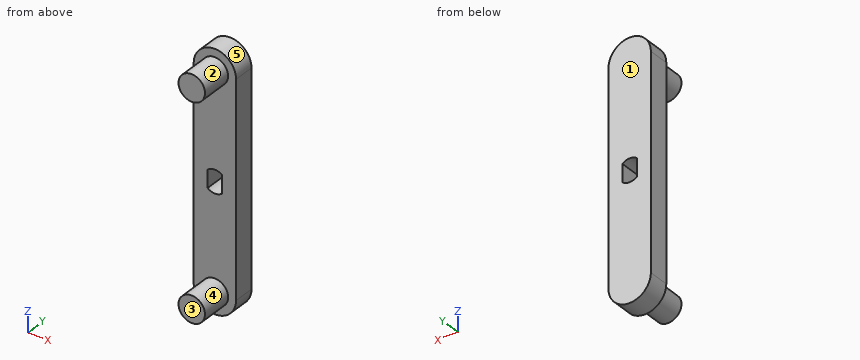
```python
from build123d import *

# Parameters (mm, degrees)
BOSS_EXTRUDE1_DEPTH = 5.08
SKETCH3_R           = 3.175
BOSS_EXTRUDE2_DEPTH = 7.62
CUT_EXTRUDE1_REACH  = 35.408


with BuildPart() as part:
    # Sketch2 → Boss-Extrude1 (new body)
    with BuildSketch(Plane(origin=(0, 0, 0), x_dir=(1, 0, 0), z_dir=(0, 1, 0))):
        with BuildLine():
            Line((-5.08, 25.4), (-5.08, -25.4))
            ThreePointArc((-5.08, -25.4), (0, -30.48), (5.08, -25.4))
            Line((5.08, -25.4), (5.08, 25.4))
            ThreePointArc((5.08, 25.4), (0, 30.48), (-5.08, 25.4))
        make_face()
    extrude(amount=BOSS_EXTRUDE1_DEPTH)

    # Sketch3 → Boss-Extrude2 (add)
    with BuildSketch(Plane(origin=(0, 0, 0), x_dir=(-1, 0, 0), z_dir=(0, -1, 0))):
        with Locations(Location((0, -25.4, 0), (0, 0, 270))):
            Circle(SKETCH3_R)
        with Locations(Location((0, 25.4, 0), (0, 0, 270))):
            Circle(SKETCH3_R)
    extrude(amount=BOSS_EXTRUDE2_DEPTH)

    # Sketch10 → Cut-Extrude1 (cut, up to next)
    with BuildSketch(Plane(origin=(0, 5.08, 0), x_dir=(1, 0, 0), z_dir=(0, 1, 0)), mode=Mode.PRIVATE) as cut_extrude1_sk1:
        with BuildLine():
            Line((-1.75, 2.121320344), (-1.75, -2.121320344))
            ThreePointArc((-1.75, -2.121320344), (0, -2.75), (1.75, -2.121320344))
            Line((1.75, -2.121320344), (1.75, 2.121320344))
            ThreePointArc((1.75, 2.121320344), (0, 2.75), (-1.75, 2.121320344))
        make_face()
    cut_extrude1_tool1 = extrude(cut_extrude1_sk1.sketch, amount=-CUT_EXTRUDE1_REACH, mode=Mode.PRIVATE) & part.part
    add(cut_extrude1_tool1.solids().sort_by_distance((0, 5.08, 0))[0], mode=Mode.SUBTRACT)


solid = part.part
```
Source: CAD feature listing. Evaluate the final solid. Frame: model axes, mm. Face numbers are marked on the shaded views. A direction names the side the tool comes from. Coordinates: 2 decimals unless noted, no trailing zeros. Write each loop counter-clockwise with the first axis right and the second up, starting at its lowest first coordinate (ties: lowest second). Pieces come first, ordered by that corner, then holes. Notation, with made-up numbers: (57, 50) -> (77, 50) arc R17 ccw to (77, 75) -> close; hole circle Ø1 at (59.25, 44). An arc over 180 degrees is marked (long way). Return JSON: item names as keys, results as strings. Group by question number.
1) Section query D-D, the plane x = 2.5. Return loops of the section in (y, z), plus the area to 3 significant figures.
2) Section query B-B, the plane y = -1. Return loops of the section in (x, z) (3 decimals).
3) Section query C-C, the plane z = 26.5. Return loops of the section in (x, y), plus the area to 3 significant figures.
4) Contact query for flat-ended pins moving along their axis: P1, Ø5, axis at x = 0, z = 7.5, coming from the -Y side; P2, Ø6, axis at x = -1.5, y = -6.5, coming from the +Z side (3 decimals). Output: stop coordinate, or through.
5) Section query A-A, the plane x = 0. Return loops of the section in (y, z) (3 decimals), plus the area to 3 significant figures.
6) Ray query, line 1 along X through (y, z) = (3.5, -2); line 2 along Y through (x, z) = (-3.75, 27.5); line 3 along Z through (x, y) = (0.25, -6.75). Return the intervals inside material, ascending.
7) Mould query, pull axis Z, two halves, no side actions, for the marked faces 3, 4 and 5. Classes: +Z half, -Z half, draft (parallel to the pull), parting line (faces both ways), or undercut.
8) Set-up query: the marked faces 1 and 2. Return all of +Z, -Z, +X, -X, +Y, -Y with unobstructed straight access to the full face (end or side cutting, diameter ignored); none if empty.
From the geometry:
{
 "1": {"outline": "(-7.62, -27.36) -> (0, -27.36) -> (0, -29.82) -> (5.08, -29.82) -> (5.08, 29.82) -> (0, 29.82) -> (0, 27.36) -> (-7.62, 27.36) -> (-7.62, 23.44) -> (0, 23.44) -> (0, -23.44) -> (-7.62, -23.44) -> close", "area": "363 mm²"},
 "2": {"outline": "circle Ø6.35 at (0, -25.4); circle Ø6.35 at (0, 25.4)"},
 "3": {"outline": "(-4.96, 0) -> (-2.98, 0) -> (-2.98, -7.62) -> (2.98, -7.62) -> (2.98, 0) -> (4.96, 0) -> (4.96, 5.08) -> (-4.96, 5.08) -> close", "area": "95.8 mm²"},
 "4": {"P1": "y = 0", "P2": "z = 28.575"},
 "5": {"outline": "(-7.62, -28.575) -> (0, -28.575) -> (0, -30.48) -> (5.08, -30.48) -> (5.08, -2.75) -> (0, -2.75) -> (0, -22.225) -> (-7.62, -22.225) -> close; (-7.62, 22.225) -> (0, 22.225) -> (0, 2.75) -> (5.08, 2.75) -> (5.08, 30.48) -> (0, 30.48) -> (0, 28.575) -> (-7.62, 28.575) -> close", "area": "379 mm²"},
 "6": {"line 1": "-5.08 to -1.75, 1.75 to 5.08", "line 2": "0 to 5.08", "line 3": "-28.57 to -22.23, 22.23 to 28.57"},
 "7": {"face 3": "draft", "face 4": "undercut", "face 5": "+Z half"},
 "8": {"face 1": "+Z, -Z, +X, -X, +Y", "face 2": "-Y"}
}
